Input: dimensioned drawing with shaded views. Units: mm. Origin: part minimum x, y, z. A direction names the side the tool comes from. Give positions to 0.01 mm unless a question says otherwise; leave off trailing zeros. Write each loop counter-clockwise with the first axis right and the second up, starting at its lowest first coordinate (ties: lowest second). Pieces come first, ordered by that corner, then holes.
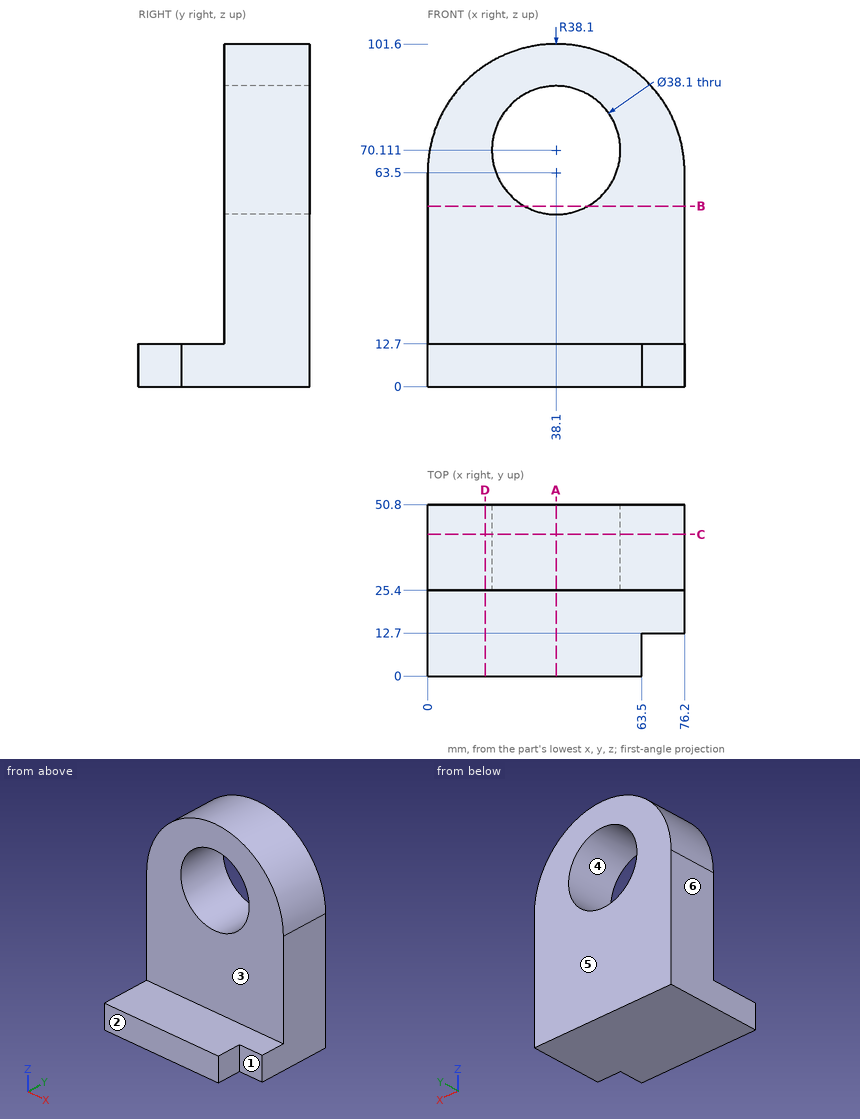
Item 1: Line query: L1, parallel to Z at x = 38.1, y = 34.25; L2, parallel to Z at x = 6.5, y = 8.5; L3, parallel to Z at x = 54, y = 46.5 (1 decimal). Output: solid intervals per line, ascending.
Found:
L1: z = 0 to 51.06, 89.16 to 101.6
L2: z = 0 to 12.7
L3: z = 0 to 59.6, 80.6 to 98.1
Item 2: Section C-C, the plane y = 42. Return the cut outline in (x, z).
Found:
outline: (0, 0) - (76.2, 0) - (76.2, 63.5) arc R38.1 ccw to (0, 63.5) - close; hole circle Ø38.1 at (38.1, 70.11)
Item 3: Section D-D, the plane x = 17. Return the cut outline in (y, z).
Found:
outline: (0, 0) - (50.8, 0) - (50.8, 95.22) - (25.4, 95.22) - (25.4, 12.7) - (0, 12.7) - close
Item 4: Pull-direction query (X, two-part tool) for the marked faces 4, 5 and 6; classes: +X half, -X half, draft (parallel to the pull), parting line (faces both ways), or undercut.
Found:
face 4: undercut
face 5: draft
face 6: -X half
Item 5: Pin query (flat end, axial travel): pin 1 Ø2 at (x, y) = (31.5, 19.5) entering from +Z; pin 2 Ø4 at (y, z) = (9, 3) entering from +X; pin 3 Ø4 at (y, z) = (41.5, 73.5) entering from -X; pin 4 Ø23 at (x, z) = (38.1, 70.11) entering from +Y. Return the tip coordinate at first contact, or that it passes through.
Found:
pin 1: stops at z = 12.7
pin 2: stops at x = 63.5
pin 3: stops at x = 0.85
pin 4: passes through
Item 6: Reachability of the marked faces 1, 2 and 3 from +Z, -Z, +X, -X, +Y, -Y: full face, straight path, thin tool, end or side. Return the list, or none.
Found:
face 1: +Z, -Z, +X, -Y
face 2: +Z, -Z, +X, -X, -Y
face 3: +Z, +X, -X, -Y
Item 7: Section B-B, the plane z = 53.5. Return the cut outline in (x, y), plus the area to 3 significant figures.
Found:
outline: (0, 25.4) - (28.77, 25.4) - (28.77, 50.8) - (0, 50.8) - close; (47.43, 25.4) - (76.2, 25.4) - (76.2, 50.8) - (47.43, 50.8) - close
area: 1,460 mm2
Item 8: Section A-A, the plane x = 38.1. Return the cut outline in (y, z).
Found:
outline: (0, 0) - (50.8, 0) - (50.8, 51.06) - (25.4, 51.06) - (25.4, 12.7) - (0, 12.7) - close; (25.4, 89.16) - (50.8, 89.16) - (50.8, 101.6) - (25.4, 101.6) - close
